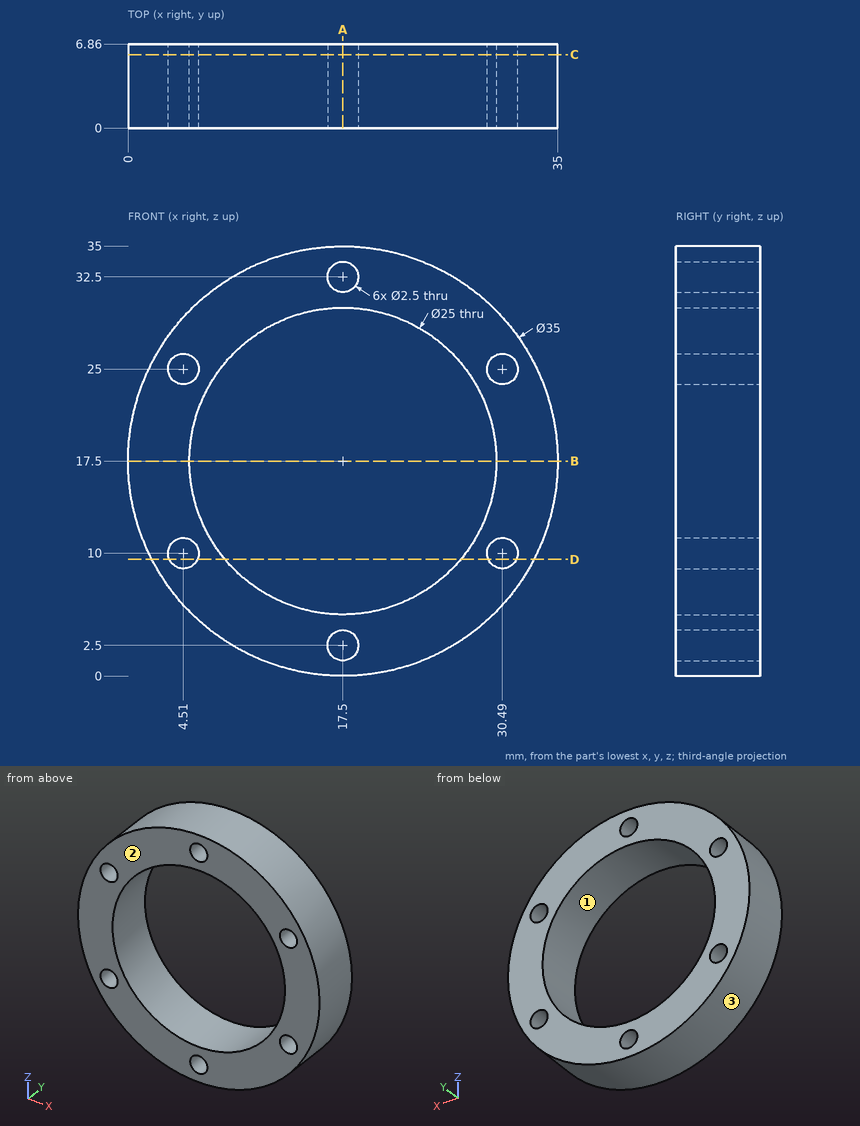
Part print with two shaded views. Sizes in mm from the minimum x, y, z corner. Coordinates: 2 decimals unless noted, no trailing zeros. Write each loop counter-clockwise with the first axis right and the second up, starting at its lowest first coordinate (ties: lowest second). Pieces come first, ordered by that corner, then holes. Notation, with made-up numbers: (-10, 53) - (47, 53) arc R29 ccw to (47, 90) - close; hole circle Ø4 at (-5.75, 27.25). An arc over 180 degrees is marked (long way). Use a Markdown table: item, result. Add a question column.
Item 1: Drill centre lines: line 1 along Z through (x, y) = (17.5, 2.25); line 2 along Z through (x, y) = (10, 5.5); line 3 along Z through (x, y) = (19, 3) (1 decimal). Where is each one in solid material? Low to high.
Item 2: Band-saw the part on D-D, the plane z = 9.5. Write the cut outline in (x, y) (1 decimal).
Item 3: Band-saw the part on C-C, the plane y = 6. Give the number of separate pieces and of enclosed holes in the cut face, and give its area (3 significant figures).
Item 4: Drop flat-ended pins along their axis: pin 1 (2 mm diameter, centred on x = 30.49, z = 25, fed in from -Y); pin 2 (3 mm diameter, centred on x = 18, z = 29, fed in from +Y); pin 3 (1.5 mm diameter, centred on y = 4, z = 8, fed in from +X) (1 decimal); pin 4 (2 mm diameter, centred on x = 20.5, y = 1, fed in from +Z) (1 decimal). Give the stop position or say it passes through.
Item 5: Two-plate mould, pull along Z, no slides. Class the marked faces 1, 2 and 3: pulls with the +Z half, pulls with the -Z half, needs draft (parallel to the pull), parting line crosses it, or undercut.
Item 6: Band-saw the part on B-B, the plane z = 17.5. Write the cut outline in (x, y).
Item 7: Band-saw the part on A-A, the plane x = 17.5. Write the cut outline in (y, z).
A:
| question | item | result |
|---|---|---|
| 1 | line 1 | z = 0 to 1.25, 3.75 to 5, 30 to 31.25, 33.75 to 35 |
| 1 | line 2 | z = 1.69 to 7.5, 27.5 to 33.31 |
| 1 | line 3 | z = 0.1 to 5.1, 29.9 to 34.9 |
| 2 | outline | (1.9, 0) - (3.4, 0) - (3.4, 6.9) - (1.9, 6.9) - close; (5.7, 0) - (7.9, 0) - (7.9, 6.9) - (5.7, 6.9) - close; (27.1, 0) - (29.3, 0) - (29.3, 6.9) - (27.1, 6.9) - close; (31.6, 0) - (33.1, 0) - (33.1, 6.9) - (31.6, 6.9) - close |
| 3 | separate pieces | 1 |
| 3 | enclosed holes | 7 |
| 3 | area | 442 mm² |
| 4 | pin 1 | passes through |
| 4 | pin 2 | stops at y = 6.86 |
| 4 | pin 3 | stops at x = 32.7 |
| 4 | pin 4 | stops at z = 34.9 |
| 5 | face 1 | undercut |
| 5 | face 2 | needs draft |
| 5 | face 3 | parting line crosses it |
| 6 | outline | (0, 0) - (5, 0) - (5, 6.86) - (0, 6.86) - close; (30, 0) - (35, 0) - (35, 6.86) - (30, 6.86) - close |
| 7 | outline | (0, 0) - (6.86, 0) - (6.86, 1.25) - (0, 1.25) - close; (0, 3.75) - (6.86, 3.75) - (6.86, 5) - (0, 5) - close; (0, 30) - (6.86, 30) - (6.86, 31.25) - (0, 31.25) - close; (0, 33.75) - (6.86, 33.75) - (6.86, 35) - (0, 35) - close |
